Work out the finished part from the listing and answer in its coordinate system (mm). A direction names the side the tool comes from. Round coordinates to 2 decimals unless told otherwise and drop trailing zeros. Write each loop counter-clockwise with the first axis right and the second up, starting at its lowest first coordinate (ties: lowest second). Pieces come first, ordered by that corner, then holes.
1. Find section A-A (x = 0). Write down the section's boundary in (y, z) (3 decimals), and give its area (3 significant figures).
2. Find section B-B (z = 0). Write down the section's boundary in (x, y) (3 decimals).
3. Determine the mould class of faces 4 (the face through (-2, 2, 0.85)), 5 (the face through (-1, 4, -1)), 6 (the face through (1.7, 3.3, 3.2)) for opening direction X: pulls with the +X half, pulls with the -X half, needs draft (parallel to the pull), parting line crosses it, or undercut.
4. Find section C-C (y = 2.35). Write down the section's boundary in (x, z) (3 decimals).
5. Flat-ended cylindrical pins translate along their axes: pin 1 Ø1.9 at (x, y) = (0, 2.5) entering from +Z (3 decimals); pin 2 Ø1.1 at (x, y) = (1.5, 1.5) entering from +Z; pin 3 Ø1.5 at (y, z) = (1, 1.5) entering from -X; pin 4 Ø0.8 at (y, z) = (2, 0.5) entering from -X. Find the tip coordinate at first contact, or state that the pin passes through.
6. A tool of negligible diameter and unlimited length cuts with its end or side. For faces 1 (the face through (2, 2, -0.85)), 2 (the face through (-1, 0, -1)), 3 (the face through (-0.37, 1.99, -2.85)), from which of +Z, -Z, +X, -X, +Y, -Y can it reach the whole face along a straight path? Write none if from no direction.
7. Straight lines are drawn through the part: probe 1 along Z at (x, y) = (0, 0.2) (3 decimals); probe 2 along Y at (x, z) = (-1.5, -2.5); probe 3 along Z at (x, y) = (-1, 2.05). For each, find the intervals that lie inside material, in ascending order.
8. Find section D-D (y = 0.4). Write down the section's boundary in (x, z) (3 decimals).
```python
from build123d import *

# Parameters (mm, degrees)
SKETCH2_R           = 3.625
BOSS_EXTRUDE1_DEPTH = 1.33333333
SKETCH6_R           = 2.875
BOSS_EXTRUDE2_DEPTH = 1.33333333
SKETCH7_R           = 3.625
BOSS_EXTRUDE3_DEPTH = 1.33333333
CUT_EXTRUDE1_DEPTH  = 4.99999999


with BuildPart() as part:
    # Sketch2 → Boss-Extrude1 (new body)
    with BuildSketch(Plane(origin=(0, 0, 0), x_dir=(1, 0, 0), z_dir=(0, 1, 0))):
        Circle(SKETCH2_R)
    extrude(amount=BOSS_EXTRUDE1_DEPTH)

    # Sketch6 → Boss-Extrude2 (add)
    with BuildSketch(Plane(origin=(0, 1.33333333, 0), x_dir=(1, 0, 0), z_dir=(0, 1, 0))):
        Circle(SKETCH6_R)
    extrude(amount=BOSS_EXTRUDE2_DEPTH)

    # Sketch7 → Boss-Extrude3 (add)
    with BuildSketch(Plane(origin=(0, 2.66666666, 0), x_dir=(1, 0, 0), z_dir=(0, 1, 0))):
        Circle(SKETCH7_R)
    extrude(amount=BOSS_EXTRUDE3_DEPTH)

    # Sketch8 → Cut-Extrude1 (cut, through all)
    with BuildSketch(Plane(origin=(0, 3.99999999, 0), x_dir=(1, 0, 0), z_dir=(0, 1, 0))):
        Polygon((-0.85, 0.85), (-0.85, 2.19089023), (0.85, 2.19089023), (0.85, 0.85), (2.19089023, 0.85), (2.19089023, -0.85), (0.85, -0.85), (0.85, -2.19089023), (-0.85, -2.19089023), (-0.85, -0.85), (-2.19089023, -0.85), (-2.19089023, 0.85), align=None)
    extrude(amount=-CUT_EXTRUDE1_DEPTH, mode=Mode.SUBTRACT)


solid = part.part
```
Worked answers:
1. outline: (0, -3.625) - (1.333, -3.625) - (1.333, -2.875) - (2.667, -2.875) - (2.667, -3.625) - (4, -3.625) - (4, -2.191) - (0, -2.191) - close; (0, 2.191) - (4, 2.191) - (4, 3.625) - (2.667, 3.625) - (2.667, 2.875) - (1.333, 2.875) - (1.333, 3.625) - (0, 3.625) - close
1. area: 9.47 mm2
2. outline: (-3.625, 0) - (-2.191, 0) - (-2.191, 4) - (-3.625, 4) - (-3.625, 2.667) - (-2.875, 2.667) - (-2.875, 1.333) - (-3.625, 1.333) - close; (2.191, 0) - (3.625, 0) - (3.625, 1.333) - (2.875, 1.333) - (2.875, 2.667) - (3.625, 2.667) - (3.625, 4) - (2.191, 4) - close
3. face 4: undercut
3. face 5: needs draft
3. face 6: parting line crosses it
4. outline: circle Ø5.75 at (0, 0); hole (-2.191, -0.85) - (-0.85, -0.85) - (-0.85, -2.191) - (0.85, -2.191) - (0.85, -0.85) - (2.191, -0.85) - (2.191, 0.85) - (0.85, 0.85) - (0.85, 2.191) - (-0.85, 2.191) - (-0.85, 0.85) - (-2.191, 0.85) - close
5. pin 1: stops at z = 3.625
5. pin 2: stops at z = 3.49
5. pin 3: stops at x = -3.55
5. pin 4: stops at x = -2.87
6. face 1: +Y, -Y
6. face 2: +Z, -Z, +X, -X, -Y
6. face 3: none
7. probe 1: z = -3.625 to -2.191, 2.191 to 3.625
7. probe 2: y = 0 to 1.33, 2.67 to 4
7. probe 3: z = -2.7 to -0.85, 0.85 to 2.7
8. outline: circle Ø7.25 at (0, 0); hole (-2.191, -0.85) - (-0.85, -0.85) - (-0.85, -2.191) - (0.85, -2.191) - (0.85, -0.85) - (2.191, -0.85) - (2.191, 0.85) - (0.85, 0.85) - (0.85, 2.191) - (-0.85, 2.191) - (-0.85, 0.85) - (-2.191, 0.85) - close
